```python
from build123d import *

# Parameters (mm, degrees)
EXTRUDE_2_DEPTH = 3


with BuildPart() as part:
    # 스케치5 → 보스-돌출2 (new body)
    with BuildSketch(Plane.XY.offset(70)):
        Polygon((54.8, -20.8), (57.8, -20.8), (57.8, 20.8), (54.8, 20.8), (54.8, 29.8), (45.8, 29.8), (45.8, 32.8), (-45.8, 32.8), (-45.8, 29.8), (-54.8, 29.8), (-54.8, 20.8), (-57.8, 20.8), (-57.8, 8.2), (-54.8, 8.2), (-54.8, -11.6), (-57.8, -11.6), (-57.8, -21), (-54.8, -21), (-54.8, -29.8), (-45.8, -29.8), (-45.8, -32.8), (45.8, -32.8), (45.8, -29.8), (54.8, -29.8), align=None)
        with BuildLine():
            Line((-17.5, 20.5), (17.5, 20.5))
            ThreePointArc((17.5, 20.5), (19.621320344, 19.621320344), (20.5, 17.5))
            Line((20.5, 17.5), (20.5, -17.5))
            ThreePointArc((20.5, -17.5), (19.621320344, -19.621320344), (17.5, -20.5))
            Line((17.5, -20.5), (-17.5, -20.5))
            ThreePointArc((-17.5, -20.5), (-19.621320344, -19.621320344), (-20.5, -17.5))
            Line((-20.5, -17.5), (-20.5, 17.5))
            ThreePointArc((-20.5, 17.5), (-19.621320344, 19.621320344), (-17.5, 20.5))
        make_face(mode=Mode.SUBTRACT)
        with BuildLine():
            Line((-29.5, 11), (-44.5, 11))
            ThreePointArc((-44.5, 11), (-48.5, 15), (-44.5, 19))
            Line((-44.5, 19), (-29.5, 19))
            ThreePointArc((-29.5, 19), (-25.5, 15), (-29.5, 11))
        make_face(mode=Mode.SUBTRACT)
        with BuildLine():
            Line((29.5, -11), (44.5, -11))
            ThreePointArc((44.5, -11), (48.5, -15), (44.5, -19))
            Line((44.5, -19), (29.5, -19))
            ThreePointArc((29.5, -19), (25.5, -15), (29.5, -11))
        make_face(mode=Mode.SUBTRACT)
        with BuildLine():
            Line((29.5, 4), (44.5, 4))
            ThreePointArc((44.5, 4), (48.5, 0), (44.5, -4))
            Line((44.5, -4), (29.5, -4))
            ThreePointArc((29.5, -4), (25.5, 0), (29.5, 4))
        make_face(mode=Mode.SUBTRACT)
        with BuildLine():
            Line((29.5, 19), (44.5, 19))
            ThreePointArc((44.5, 19), (48.5, 15), (44.5, 11))
            Line((44.5, 11), (29.5, 11))
            ThreePointArc((29.5, 11), (25.5, 15), (29.5, 19))
        make_face(mode=Mode.SUBTRACT)
        with BuildLine():
            Line((-29.5, -19), (-44.5, -19))
            ThreePointArc((-44.5, -19), (-48.5, -15), (-44.5, -11))
            Line((-44.5, -11), (-29.5, -11))
            ThreePointArc((-29.5, -11), (-25.5, -15), (-29.5, -19))
        make_face(mode=Mode.SUBTRACT)
        with BuildLine():
            Line((-29.5, -4), (-44.5, -4))
            ThreePointArc((-44.5, -4), (-48.5, 0), (-44.5, 4))
            Line((-44.5, 4), (-29.5, 4))
            ThreePointArc((-29.5, 4), (-25.5, 0), (-29.5, -4))
        make_face(mode=Mode.SUBTRACT)
    extrude(amount=-EXTRUDE_2_DEPTH)


solid = part.part
```
Check sheet for the modelled part. Datum: model origin and axes. Units: mm. A direction names the side the tool comes from. Coordinates: 2 decimals unless noted, no trailing zeros. Loops run counter-clockwise (first coordinate to the right, second up) from the corner with the lowest first, then second, coordinate; pieces in that order, holes last. Notation, with made-up numbers: M 39.5,77 L 52.5,77 A23 ccw 52.5,114 Z; hole C -36,40.5 d9. An arc over 180 degrees is marked long. Answer as a JSON object with one key per item and string values.
1. Sectioned sample at C-C on y = 7. Record the cut outline in (x, z), and give its area (3 significant figures).
Outcome:
{"outline": "M -54.8,67 L -20.5,67 L -20.5,70 L -54.8,70 Z; M 20.5,67 L 57.8,67 L 57.8,70 L 20.5,70 Z", "area": "215 mm²"}
2. Access from +Z, -Z, +X, -X, +Y, -Y to the whole of each face (thin tool, end or side, straight path). Record for faces 4 (the cylindrical face through (-19.64, 19.6, 68.52)), 5 (the flat face through (1, 32.8, 69)).
Outcome:
{"face 4": "+Z, -Z", "face 5": "+Z, -Z, +X, -X, +Y"}
3. Sectioned sample at B-B on x = -4.5. Record the cut outline in (y, z), and give its area (3 significant figures).
Outcome:
{"outline": "M -32.8,67 L -20.5,67 L -20.5,70 L -32.8,70 Z; M 20.5,67 L 32.8,67 L 32.8,70 L 20.5,70 Z", "area": "73.8 mm²"}
4. Sectioned sample at D-D on x = -43. Record the cut outline in (y, z), and give its area (3 significant figures).
Outcome:
{"outline": "M -32.8,67 L -19,67 L -19,70 L -32.8,70 Z; M -11,67 L -4,67 L -4,70 L -11,70 Z; M 4,67 L 11,67 L 11,70 L 4,70 Z; M 19,67 L 32.8,67 L 32.8,70 L 19,70 Z", "area": "125 mm²"}
5. Sectioned sample at A-A on y = 15. Record the cut outline in (x, z), and give its area (3 significant figures).
Outcome:
{"outline": "M -57.8,67 L -48.5,67 L -48.5,70 L -57.8,70 Z; M -25.5,67 L -20.5,67 L -20.5,70 L -25.5,70 Z; M 20.5,67 L 25.5,67 L 25.5,70 L 20.5,70 Z; M 48.5,67 L 57.8,67 L 57.8,70 L 48.5,70 Z", "area": "85.8 mm²"}
6. Scan lines: L1, parallel to Y at x = -30, z = 69; L2, parallel to X at y = -4.5, z = 67.45; L3, parallel to Y at x = 14.5, z = 69.15. Record each from-to range of solid material in increasing order. Write a range as from..to.
Outcome:
{"L1": "-32.8..-19, -11..-4, 4..11, 19..32.8", "L2": "-54.8..-20.5, 20.5..57.8", "L3": "-32.8..-20.5, 20.5..32.8"}
7. Release check for a two-part mould opening along X. For faces 1 (the flat face through (37, 4, 69)), 2 (the flat face through (-56, 8.2, 69)), 3 (the flat face through (-54.8, -2, 69)) record: pulls with the +X half, pulls with the -X half, needs draft (parallel to the pull), parting line crosses it, or undercut.
Outcome:
{"face 1": "undercut", "face 2": "needs draft", "face 3": "pulls with the -X half"}
8. Depth check by flat-ended pin: P1, Ø0.9, axis at x = 56, z = 69, coming from the +Y side; P2, Ø1.5, axis at x = -51, z = 68, coming from the +Y side; P3, Ø0.9, axis at x = -55.5, z = 68.5, coming from the -Y side. Enter the tip coordinate at first touch or a pass-through.
Outcome:
{"P1": "y = 20.8", "P2": "y = 29.8", "P3": "y = -21"}
